Can you work these out from the model? Positions are in its coordinate system, mm. A direction names the side the tool comes from. Coordinates: 2 decimals unless noted, no trailing zeros. Write each loop counter-clockwise with the first axis right and the second up, starting at its lowest first coordinate (ties: lowest second). Pieces come first, ordered by that corner, then holes. Notation, with made-up numbers: (42.5, 18.5) -> (91.5, 18.5) arc R31 cw to (91.5, 55.5) -> close; hole circle Ø8 at (78, 35). An arc over 180 degrees is marked (long way). Answer as CSV lines item,"result". Start each with the question number.
```python
from build123d import *

# Parameters (mm, degrees)
F0_W     = 35
F0_H     = 8.31089
F1_DEPTH = 6.35
F2_W     = 6.9
F2_H     = 5.85
F3_DEPTH = 6.35


# Not quite as in the source:
# - a length typed as a fraction of an inch, garbled in the dataset ("3 / 203.2 mm" for 3/8 in), is restored


with BuildPart() as f1:
    # F0 (on Front) → F1 (new body)
    with BuildSketch(Plane.XZ):
        with BuildLine():
            ThreePointArc((17.5, 9.6824583655), (19.364916731, 5), (20, 0))
            ThreePointArc((20, 0), (19.364916731, -5), (17.5, -9.6824583655))
            Line((17.5, -9.6824583655), (17.5, -22))
            Line((17.5, -22), (22, -22))
            Line((22, -22), (22, 22))
            Line((22, 22), (17.5, 22))
            Line((17.5, 22), (17.5, 9.6824583655))
        make_face()
        with BuildLine():
            ThreePointArc((-17.5, -9.6824583655), (-20, 0), (-17.5, 9.6824583655))
            Line((-17.5, 9.6824583655), (-17.5, 22))
            Line((-17.5, 22), (-22, 22))
            Line((-22, 22), (-22, -22))
            Line((-22, -22), (-17.5, -22))
            Line((-17.5, -22), (-17.5, -9.6824583655))
        make_face()
        with Locations((0, 26.155445)):
            Rectangle(F0_W, F0_H)
        Polygon((17.5, 30.31089), (17.5, 22), (22, 22), align=None)
        Polygon((22, -22), (17.5, -22), (17.5, -30.31089), align=None)
        with Locations((0, -26.155445)):
            Rectangle(F0_W, F0_H)
        Polygon((-22, 22), (-17.5, 22), (-17.5, 30.31089), align=None)
        Polygon((-17.5, -30.31089), (-17.5, -22), (-22, -22), align=None)
        with BuildLine():
            ThreePointArc((-17.5, 9.6824583655), (0, 20), (17.5, 9.6824583655))
            Line((17.5, 9.6824583655), (17.5, 22))
            Line((17.5, 22), (-17.5, 22))
            Line((-17.5, 22), (-17.5, 9.6824583655))
        make_face()
        with BuildLine():
            Line((17.5, -22), (17.5, -9.6824583655))
            ThreePointArc((17.5, -9.6824583655), (0, -20), (-17.5, -9.6824583655))
            Line((-17.5, -9.6824583655), (-17.5, -22))
            Line((-17.5, -22), (17.5, -22))
        make_face()
    extrude(amount=F1_DEPTH)

    # F2 (on face) → F3 (join)
    with BuildSketch(Plane.XZ.offset(6.35)):
        with Locations((-7.2, 33.23589)):
            Rectangle(F2_W, F2_H)
        with Locations((7.2, 33.23589)):
            Rectangle(F2_W, F2_H)
        with Locations((-7.2, -33.23589)):
            Rectangle(F2_W, F2_H)
        with Locations((7.2, -33.23589)):
            Rectangle(F2_W, F2_H)
    extrude(amount=-F3_DEPTH)


solid = f1.part
```
Q1. Imagine slicing it at B-B (y = -3.25). Write out the boundary of the cut face in (x, z).
Q2. Which directions (+Z, -Z, +X, -X, +Y, -Y) give clear straight access to the entire face, cutting with the end or side of a thin tool? Please do faces 5 (the face through (3.75, -3, -33)), 6 (the face through (-14, -3, -30.311)), 7 (the face through (-14, -3, 30.311)).
Q3. For pin 1 (1.9 mm diameter, centred on x = -1.5, y = -3.5, fed in from -Z); pin 2 (3 mm diameter, centred on y = -3, z = -34.5, fed in from +X); pin 3 (1.9 mm diameter, centred on x = -13.5, y = -2.5, fed in from +Z), each with a flat end and sliding along its axis, tell me the tip position at first contact or that it passes through.
Q4. Imagine slicing it at D-D (z = -29.5). Write out the boundary of the cut face in (x, y).
Q5. If we mould it in two halves opening along X, with no side actions, what happens to faces 1 (the face through (-10.65, -3, 33)), 2 (the face through (14, -3, 30.311)), 3 (the face through (0, -3, -30.311)), 4 (the face through (-3.75, -3, 33))? For each: released by +X, released by -X, zero draft, split by the parting line, or undercut.
Q6. Imagine slicing it at C-C (z = -1). Write out the boundary of the cut face in (x, y), then the cut area to 3 significant figures.
Q7. I need wall thicknesses on L1, parallel to Z at x = 0.5, y = -5.5; L2, parallel to Z at x = 13, y = -5; L3, parallel to X at y = -4.5, z = -6. Which ranges of each line are inside material? Lowest first, please.
Q8. Imagine slicing it at A-A (x = -12). Write out the boundary of the cut face in (y, z), then the cut area to 3 significant figures.
Entries:
1,outline,"(-22, -22) -> (-17.5, -30.31) -> (-10.65, -30.31) -> (-10.65, -36.16) -> (-3.75, -36.16) -> (-3.75, -30.31) -> (3.75, -30.31) -> (3.75, -36.16) -> (10.65, -36.16) -> (10.65, -30.31) -> (17.5, -30.31) -> (22, -22) -> (22, 22) -> (17.5, 30.31) -> (10.65, 30.31) -> (10.65, 36.16) -> (3.75, 36.16) -> (3.75, 30.31) -> (-3.75, 30.31) -> (-3.75, 36.16) -> (-10.65, 36.16) -> (-10.65, 30.31) -> (-17.5, 30.31) -> (-22, 22) -> close; hole circle Ø40 at (0, 0)"
2,face 5,"-Z, +Y, -Y"
2,face 6,"-Z, -X, +Y, -Y"
2,face 7,"+Z, -X, +Y, -Y"
3,pin 1,"z = -30.31"
3,pin 2,"x = 10.65"
3,pin 3,"z = 30.31"
4,outline,"(-17.94, -6.35) -> (17.94, -6.35) -> (17.94, 0) -> (-17.94, 0) -> close"
5,face 1,"released by -X"
5,face 2,"zero draft"
5,face 3,"undercut"
5,face 4,"undercut"
6,outline,"(-22, -6.35) -> (-19.97, -6.35) -> (-19.97, 0) -> (-22, 0) -> close; (19.97, -6.35) -> (22, -6.35) -> (22, 0) -> (19.97, 0) -> close"
6,area,"25.7 mm2"
7,L1,"-30.31 to -19.99, 19.99 to 30.31"
7,L2,"-30.31 to -15.2, 15.2 to 30.31"
7,L3,"-22 to -19.08, 19.08 to 22"
8,outline,"(-6.35, -30.31) -> (0, -30.31) -> (0, -16) -> (-6.35, -16) -> close; (-6.35, 16) -> (0, 16) -> (0, 30.31) -> (-6.35, 30.31) -> close"
8,area,"182 mm2"
